Design review of the part built by this model. Coordinates are the model's own, in mm. Face numbers are marked on the shaded views. A direction names the side the tool comes from. Coordinates: 2 decimals unless noted, no trailing zeros. Write each loop counter-clockwise with the first axis right and the second up, starting at its lowest first coordinate (ties: lowest second). Pieces come first, ordered by that corner, then holes.
Q1. Take a section at D-D (z = 5.75). Give the boundary of the cut face in (x, y), and give its area (3 significant figures).
Q2. Take a section at C-C (y = 2.5). Give the boundary of the cut face in (x, z).
Q3. Take a section at A-A (z = 3). Give the boundary of the cut face in (x, y), and give its area (3 significant figures).
Q4. Take a section at B-B (x = 4.5). Give the boundary of the cut face in (y, z).
Q5. Mouldability with a two-part tool opening along X and no side actions: class the marked faces 3, 4 and 5 as pulls with the +X half, pulls with the -X half, needs draft (parallel to the pull), parting line crosses it, or undercut.
Q6. For probe 1 along Y at (x, z) = (-21, 2); probe 2 along X at (y, z) = (15.5, 4.25); probe 3 along X at (y, z) = (-2.5, 2.75), list the stretches that pass through material, from the lowest coordinate up.
Q7. Machinability: for the marked faces 1 and 2, which of the approach directions +Z, -Z, +X, -X, +Y, -Y give a long, thin tool a straight path to every point of the face, cutting with its end or side? Answer none if there is none.
Q8. Insertion check: pin 1 (5 mm diameter, centred on x = 1, y = 6, fed in from -Z). The pin has a flat end and moves straight along its axis. Give the tip position at first contact, or say it passes through.
```python
from build123d import *

# Parameters (mm, degrees)
SKETCH_R             = 2.7
PAD_DEPTH            = 9
SKETCH_MIRRORED_2_R  = 2.7
PAD_MIRRORED_2_DEPTH = 9
POCKET_DEPTH         = 4


with BuildPart() as part:
    # Sketch → Pad (new body)
    with BuildSketch(Plane.XY):
        with BuildLine():
            ThreePointArc((0, -5.2), (3.676955, -3.676955), (5.2, 0))
            Line((5.2, 0), (27.7, 0))
            Line((27.7, 0), (27.7, -15.5))
            ThreePointArc((21, -22.2), (25.737615, -20.237615), (27.7, -15.5))
            Line((21, -22.2), (0, -22.2))
            Line((0, -22.2), (0, -5.2))
        make_face()
        with Locations((21, -15.5)):
            Circle(SKETCH_R, mode=Mode.SUBTRACT)
    pad = extrude(amount=PAD_DEPTH)

    # Sketch Mirrored 2 → Pad Mirrored 2 (add)
    with BuildSketch(Plane(origin=(0, 0, 0), x_dir=(-1, 0, 0), z_dir=(0, 0, -1))):
        with BuildLine():
            ThreePointArc((0, -5.2), (3.676955, -3.676955), (5.2, 0))
            Line((5.2, 0), (27.7, 0))
            Line((27.7, 0), (27.7, -15.5))
            ThreePointArc((21, -22.2), (25.737615, -20.237615), (27.7, -15.5))
            Line((21, -22.2), (0, -22.2))
            Line((0, -22.2), (0, -5.2))
        make_face()
        with Locations((21, -15.5)):
            Circle(SKETCH_MIRRORED_2_R, mode=Mode.SUBTRACT)
    pad_mirrored_2 = extrude(amount=-PAD_MIRRORED_2_DEPTH)

    # Mirrored001: Pad, Pad Mirrored 2 across Sketch H_Axis
    add(pad.mirror(Plane.ZX))
    add(pad_mirrored_2.mirror(Plane.ZX))

    # Sketch001 → Pocket (cut)
    with BuildSketch(Plane.XY):
        Polygon((8.5, 4.907477), (0, 9.814955), (-8.5, 4.907477), (-8.5, -4.907477), (0, -9.814955), (8.5, -4.907477), align=None)
    extrude(amount=POCKET_DEPTH, mode=Mode.SUBTRACT)


solid = part.part
```
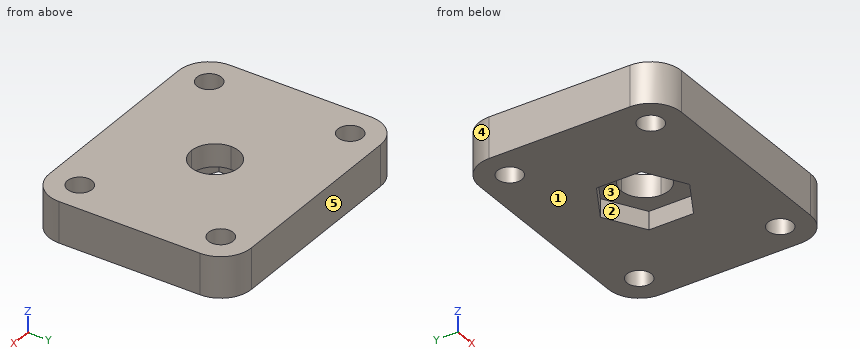
Response:
1. outline: (-27.7, -15.5) arc R6.7 ccw to (-21, -22.2) - (21, -22.2) arc R6.7 ccw to (27.7, -15.5) - (27.7, 15.5) arc R6.7 ccw to (21, 22.2) - (-21, 22.2) arc R6.7 ccw to (-27.7, 15.5) - close; hole circle Ø5.4 at (-21, -15.5); hole circle Ø5.4 at (-21, 15.5); hole (-5.2, 0) arc R5.2 ccw to (0, -5.2) arc R5.2 ccw to (5.2, 0) arc R5.2 ccw to (0, 5.2) arc R5.2 ccw to start; hole circle Ø5.4 at (21, -15.5); hole circle Ø5.4 at (21, 15.5)
1. area: 2,240 mm2
2. outline: (-27.7, 0) - (-8.5, 0) - (-8.5, 4) - (-4.56, 4) - (-4.56, 9) - (-27.7, 9) - close; (4.56, 4) - (8.5, 4) - (8.5, 0) - (27.7, 0) - (27.7, 9) - (4.56, 9) - close
3. outline: (-27.7, -15.5) arc R6.7 ccw to (-21, -22.2) - (21, -22.2) arc R6.7 ccw to (27.7, -15.5) - (27.7, 15.5) arc R6.7 ccw to (21, 22.2) - (-21, 22.2) arc R6.7 ccw to (-27.7, 15.5) - close; hole circle Ø5.4 at (-21, -15.5); hole circle Ø5.4 at (-21, 15.5); hole (-8.5, -4.91) - (0, -9.81) - (8.5, -4.91) - (8.5, 4.91) - (0, 9.81) - (-8.5, 4.91) - close; hole circle Ø5.4 at (21, -15.5); hole circle Ø5.4 at (21, 15.5)
3. area: 2,080 mm2
4. outline: (-22.2, 0) - (-7.22, 0) - (-7.22, 4) - (-2.61, 4) - (-2.61, 9) - (-22.2, 9) - close; (2.61, 4) - (7.22, 4) - (7.22, 0) - (22.2, 0) - (22.2, 9) - (2.61, 9) - close
5. face 3: undercut
5. face 4: pulls with the -X half
5. face 5: needs draft
6. probe 1: y = -22.2 to -18.2, -12.8 to 12.8, 18.2 to 22.2
6. probe 2: x = -27.7 to -23.7, -18.3 to 18.3, 23.7 to 27.7
6. probe 3: x = -27.7 to -8.5, 8.5 to 27.7
7. face 1: -Z, +X, -X, +Y, -Y
7. face 2: -Z
8. pin 1: stops at z = 4
